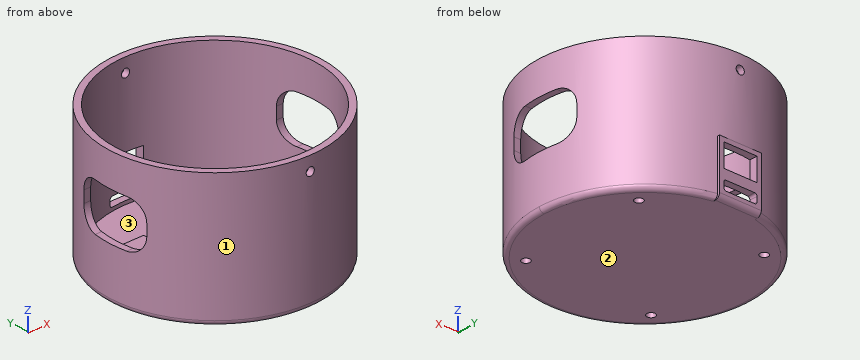
from build123d import *

# Parameters (mm, degrees)
SKETCH_R        = 45.5
PAD_DEPTH       = 56
SKETCH001_R     = 42.75
POCKET_DEPTH    = 54
SKETCH002_W     = 20
SKETCH002_H     = 15
PAD001_DEPTH    = 12
SKETCH003_W     = 30
SKETCH003_H     = 20
POCKET001_DEPTH = 60
SKETCH004_W     = 18
SKETCH004_H     = 2.55
PAD002_DEPTH    = 23
SKETCH005_W     = 14.3
SKETCH005_H     = 4
SKETCH005_H_2   = 9.7
POCKET002_DEPTH = 5
SKETCH007_R     = 1.75
POCKET003_DEPTH = 60
FILLET_R        = 2
FILLET001_R     = 2
FILLET002_R     = 1
FILLET003_R     = 7.5
SKETCH006_R     = 1.75
POCKET004_DEPTH = 2.5


with BuildPart() as part:
    # Sketch → Pad (new body)
    with BuildSketch(Plane.XY):
        Circle(SKETCH_R)
    extrude(amount=PAD_DEPTH)

    # Sketch001 (on Face3 of Pad) → Pocket (cut)
    with BuildSketch(Plane.XY.offset(56)):
        Circle(SKETCH001_R)
    extrude(amount=-POCKET_DEPTH, mode=Mode.SUBTRACT)

    # Sketch002 (on Face5 of Pocket) → Pad001 (join)
    with BuildSketch(Plane.XY.offset(2)):
        with Locations((-34, 0)):
            Rectangle(SKETCH002_W, SKETCH002_H)
        with Locations((34, 0)):
            Rectangle(SKETCH002_W, SKETCH002_H)
    extrude(amount=PAD001_DEPTH)

    # Sketch003 → Pocket001 (cut, symmetric)
    with BuildSketch(Plane.YZ):
        with Locations((0, 32)):
            Rectangle(SKETCH003_W, SKETCH003_H)
    extrude(amount=POCKET001_DEPTH, both=True, mode=Mode.SUBTRACT)

    # Sketch004 → Pad002 (join)
    with BuildSketch(Plane.XY):
        with Locations((0, 44.275)):
            Rectangle(SKETCH004_W, SKETCH004_H)
    extrude(amount=PAD002_DEPTH)

    # Sketch005 (on Face15 of Pad002) → Pocket002 (cut)
    with BuildSketch(Plane(origin=(0, 45.55, 0), x_dir=(-1, 0, 0), z_dir=(0, 1, 0))):
        with Locations((0, 5.5)):
            Rectangle(SKETCH005_W, SKETCH005_H)
        with Locations((0, 16.35)):
            Rectangle(SKETCH005_W, SKETCH005_H_2)
    extrude(amount=-POCKET002_DEPTH, mode=Mode.SUBTRACT)

    # Sketch007 → Pocket003 (cut, symmetric)
    with BuildSketch(Plane.XZ):
        with Locations((0, 50)):
            Circle(SKETCH007_R)
    extrude(amount=POCKET003_DEPTH, both=True, mode=Mode.SUBTRACT)

    # Fillet
    fillet_edges = [part.edges().sort_by_distance(p)[0] for p in [
        (35.211859, 28.816228, 0),
        (-28.816228, -35.211859, 0),
    ]]
    fillet(fillet_edges, radius=FILLET_R)

    # Fillet001
    fillet001_edges = [part.edges().sort_by_distance(p)[0] for p in [
        (0, 45.55, 0),
    ]]
    fillet(fillet001_edges, radius=FILLET001_R)

    # Fillet002
    fillet002_edges = [part.edges().sort_by_distance(p)[0] for p in [
        (7.15, 43.848918, 3.5),
        (7.15, 43.848918, 7.5),
        (-7.15, 43.848918, 7.5),
        (-7.15, 43.848918, 3.5),
    ]]
    fillet(fillet002_edges, radius=FILLET002_R)

    # Fillet003
    fillet003_edges = [part.edges().sort_by_distance(p)[0] for p in [
        (41.494196, -15, 42),
        (41.494196, 15, 42),
        (41.494196, 15, 22),
        (41.494196, -15, 22),
        (-41.494196, 15, 42),
        (-41.494196, -15, 42),
        (-41.494196, 15, 22),
        (-41.494196, -15, 22),
    ]]
    fillet(fillet003_edges, radius=FILLET003_R)

    # Sketch006 → Pocket004 (cut, symmetric)
    with BuildSketch(Plane.XY):
        with Locations((-27, 27)):
            Circle(SKETCH006_R)
        with Locations((27, 27)):
            Circle(SKETCH006_R)
        with Locations((-27, -27)):
            Circle(SKETCH006_R)
        with Locations((27, -27)):
            Circle(SKETCH006_R)
    extrude(amount=POCKET004_DEPTH, both=True, mode=Mode.SUBTRACT)


solid = part.part
Geometry check sheet. Reference: the model listing, model coordinates, mm. Face numbers are marked on the shaded views. Give positions to 0.01 mm unless a question says otherwise; leave off trailing zeros. Loops run counter-clockwise (first coordinate to the right, second up) from the corner with the lowest first, then second, coordinate; pieces in that order, holes last. Notation, with made-up numbers: M 71.5,-23 L 88.5,-23 A18 cw 88.5,8 Z; hole C 46,21 d7. An arc over 180 degrees is marked long. Answer as a JSON object with one key per item and string values. Group by question number.
Item 1: Gauge pin test, flat ends, axial feed: pin 1 (12 mm diameter, centred on x = 16, y = 29.5, fed in from +Z); pin 2 (6 mm diameter, centred on x = -32, z = 5, fed in from -Y); pin 3 (1.5 mm diameter, centred on x = -31.5, y = -35.5, fed in from +Z); pin 4 (12 mm diameter, centred on x = 33, y = 0, fed in from +Z). Record the tip position at first contact, or that the pin passes through.
Item 2: Sectioned sample at C-C on y = -3. Give the number of separate pieces and of enclosed holes in the cut face, plus the area to 3 significant figures.
Item 3: Sectioned sample at B-B on z = 18. Record the boundary of the cut face in (x, y), plus the area to 3 significant figures.
Item 4: Material ranges on L1, parallel to X at y = 27, z = 1.35; L2, parallel to X at y = 0, z = 13.5; L3, parallel to Y at x = -27, z = 0.6, recorded low to high.
Item 5: Mould release check, pull along X, two halves, no side actions. Record for the marked faces 1, 2 and 3: pulls with the +X half, pulls with the -X half, needs draft (parallel to the pull), parting line crosses it, or undercut.
Findings below:
{
 "1": {"pin 1": "z = 2", "pin 2": "y = -35.06", "pin 3": "through", "pin 4": "z = 14"},
 "2": {"separate pieces": "3", "enclosed holes": "0", "area": "815 mm2"},
 "3": {"outline": "M -9,44.6 A45.5 ccw long 9,44.6 L 9,45.55 L 7.15,45.55 L 7.15,42.15 A42.75 cw long -7.15,42.15 L -7.15,45.55 L -9,45.55 Z", "area": "726 mm2"},
 "4": {"L1": "-36.49 to -28.75, -25.25 to 25.25, 28.75 to 36.49", "L2": "-45.5 to -24, 24 to 45.5", "L3": "-35.91 to -28.75, -25.25 to 25.25, 28.75 to 35.91"},
 "5": {"face 1": "parting line crosses it", "face 2": "needs draft", "face 3": "undercut"}
}
